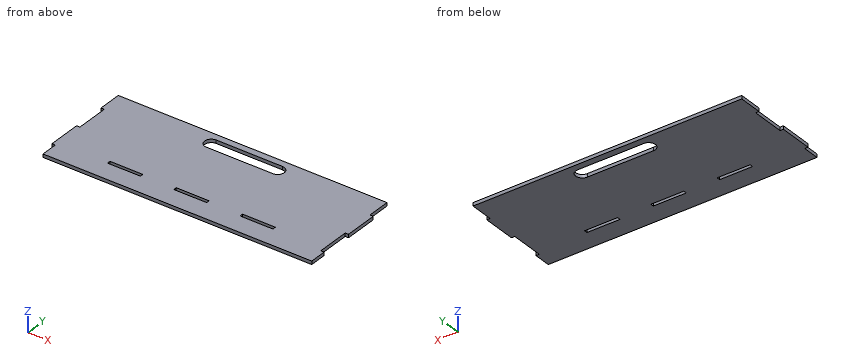
from build123d import *

# Parameters (mm, degrees)
SKIZZE1_W                       = 410
SKIZZE1_H                       = 300
AUFSATZ_LINEAR_AUSTRAGEN1_DEPTH = 5
SKIZZE2_W                       = 46.676040128
SKIZZE2_H                       = 49.6
SCHNITT_LINEAR_AUSTRAGEN1_DEPTH = 5
LINEARES_MUSTER1_COUNT          = 4
LINEARES_MUSTER1_PITCH          = 99.9
SKIZZE3_W                       = 27.663601369
SKIZZE3_H                       = 49.6
SCHNITT_LINEAR_AUSTRAGEN2_DEPTH = 5
LINEARES_MUSTER2_COUNT          = 3
LINEARES_MUSTER2_PITCH          = 99.9
SKIZZE4_W                       = 49.6
SKIZZE4_H                       = 5
SCHNITT_LINEAR_AUSTRAGEN3_DEPTH = 5
LINEARES_MUSTER3_COUNT          = 3
LINEARES_MUSTER3_PITCH          = 99.9
SCHNITT_LINEAR_AUSTRAGEN4_DEPTH = 5


with BuildPart() as part:
    # Skizze1 → Aufsatz-Linear austragen1 (new body)
    with BuildSketch(Plane.XY):
        with Locations((205, 150)):
            Rectangle(SKIZZE1_W, SKIZZE1_H)
    extrude(amount=AUFSATZ_LINEAR_AUSTRAGEN1_DEPTH)

    # Skizze2 → Schnitt-Linear austragen1 (cut)
    with BuildSketch(Plane.XY.offset(5)):
        with Locations((-18.338020064, 299.85)):
            Rectangle(SKIZZE2_W, SKIZZE2_H)
    schnitt_linear_austragen1 = extrude(amount=-SCHNITT_LINEAR_AUSTRAGEN1_DEPTH, mode=Mode.SUBTRACT)

    # Lineares Muster1: Schnitt-Linear austragen1 ×4
    with Locations(*[(0, -i * LINEARES_MUSTER1_PITCH, 0) for i in range(1, LINEARES_MUSTER1_COUNT)]):
        add(schnitt_linear_austragen1, mode=Mode.SUBTRACT)

    # Skizze3 → Schnitt-Linear austragen2 (cut)
    with BuildSketch(Plane.XY.offset(5)):
        with Locations((418.831800685, 249.9)):
            Rectangle(SKIZZE3_W, SKIZZE3_H)
    schnitt_linear_austragen2 = extrude(amount=-SCHNITT_LINEAR_AUSTRAGEN2_DEPTH, mode=Mode.SUBTRACT)

    # Lineares Muster2: Schnitt-Linear austragen2 ×3
    with Locations(*[(0, -i * LINEARES_MUSTER2_PITCH, 0) for i in range(1, LINEARES_MUSTER2_COUNT)]):
        add(schnitt_linear_austragen2, mode=Mode.SUBTRACT)

    # Skizze4 → Schnitt-Linear austragen3 (cut)
    with BuildSketch(Plane.XY.offset(5)):
        with Locations((104.75, 32.5)):
            Rectangle(SKIZZE4_W, SKIZZE4_H)
    schnitt_linear_austragen3 = extrude(amount=-SCHNITT_LINEAR_AUSTRAGEN3_DEPTH, mode=Mode.SUBTRACT)

    # Lineares Muster3: Schnitt-Linear austragen3 ×3
    with Locations(*[(i * LINEARES_MUSTER3_PITCH, 0, 0) for i in range(1, LINEARES_MUSTER3_COUNT)]):
        add(schnitt_linear_austragen3, mode=Mode.SUBTRACT)

    # Skizze5 → Schnitt-Linear austragen4 (cut)
    with BuildSketch(Plane.XY.offset(5)):
        Polygon((0, 160), (405, 160), (496.663114114, 346.337546914), (-27.8257996, 333.824324496), (-27.8257996, 200.492217914), align=None)
        with BuildLine():
            Line((155, 150), (255, 150))
            ThreePointArc((255, 150), (265, 140), (255, 130))
            Line((255, 130), (155, 130))
            ThreePointArc((155, 130), (145, 140), (155, 150))
        make_face()
    extrude(amount=-SCHNITT_LINEAR_AUSTRAGEN4_DEPTH, mode=Mode.SUBTRACT)


solid = part.part
Could you check a few things on this model? Use its own coordinates, in mm. Give positions to 0.01 mm unless a question says otherwise; leave off trailing zeros. Order: outer loops, then holes, each group sorted by start corner. A loop starts at its lowest first (then second) coordinate and runs counter-clockwise, first axis right, second up.
Item 1: If we section it at C-C, the plane x = 206: Write out the boundary of the cut face in (y, z), plus the area to 3 significant figures.
Item 2: I need wall thicknesses on line 1 (Y direction, x = 215.5, z = 0.45); line 2 (Y direction, x = 96.5, z = 1.15); line 3 (X direction, y = 106, z = 2.75). Which ranges of each line are inside material? Lowest first, please.
Item 3: I'm going to push flat-ended pins straight in: pin 1 (1.5 mm diameter, centred on y = 142, z = 4, fed in from +X); pin 2 (2.5 mm diameter, centred on x = 408, z = 2.5, fed in from +Y); pin 3 (1.5 mm diameter, centred on x = 3, z = 3, fed in from -Y). Where does each tip first touch, or does it pass through?
Item 4: If we section it at A-A, the plane y = 140: Write out the boundary of the cut face in (x, z), plus the area to 4 significant figures.
Item 5: If we section it at B-B, the plane z = 3: Count the separate pieces of the cut face and the enclosed holes in it, plus the area to 3 significant figures.
Item 6: If we section it at D-D, the plane x = 314.5: Write out the boundary of the cut face in (y, z).
Values:
1. outline: (0, 0) - (30, 0) - (30, 5) - (0, 5) - close; (35, 0) - (130, 0) - (130, 5) - (35, 5) - close; (150, 0) - (160, 0) - (160, 5) - (150, 5) - close
1. area: 675 mm2
2. line 1: y = 0 to 30, 35 to 130, 150 to 160
2. line 2: y = 0 to 30, 35 to 160
2. line 3: x = 5 to 410
3. pin 1: stops at x = 405
3. pin 2: stops at y = 125.2
3. pin 3: stops at y = 24.95
4. outline: (0, 0) - (145, 0) - (145, 5) - (0, 5) - close; (265, 0) - (405, 0) - (405, 5) - (265, 5) - close
4. area: 1,425 mm2
5. separate pieces: 1
5. enclosed holes: 4
5. area: 61,700 mm2
6. outline: (0, 0) - (30, 0) - (30, 5) - (0, 5) - close; (35, 0) - (160, 0) - (160, 5) - (35, 5) - close
